```python
from build123d import *

# Parameters (mm, degrees)
F0_R     = 15
F1_DEPTH = 50
F2_R     = 25
F3_DEPTH = 5
F4_R     = 3
F5_DEPTH = 60


with BuildPart() as f1:
    # F0 (on Top) → F1 (new body)
    with BuildSketch(Plane.XY):
        Circle(F0_R)
    extrude(amount=F1_DEPTH)

    # F2 (on Top) → F3 (join)
    with BuildSketch(Plane.XY):
        Circle(F2_R)
    extrude(amount=F3_DEPTH)


with BuildPart() as f5:
    # F4 (on Top) → F5 (new body)
    with BuildSketch(Plane.XY):
        Circle(F4_R)
    extrude(amount=F5_DEPTH)


with BuildPart() as f1_1:
    add(f1.part)

    # F6: cut F5
    add(f5.part, mode=Mode.SUBTRACT)


solid = f1_1.part
```
Input: part model. Units: mm. Frame: model coordinates. Round coordinates to 2 decimals unless told otherwise and drop trailing zeros. Loops run counter-clockwise (first coordinate to the right, second up) from the corner with the lowest first, then second, coordinate; pieces in that order, holes last. Notation, with made-up numbers: (16, -5.75) -> (27, -5.75) arc R30 ccw to (27, 20.25) -> close; hole circle Ø11 at (13, 72.25). An arc over 180 degrees is marked (long way). One line per item, written item: value.
(1) Pin query (flat end, axial travel): pin 1 (6 mm diameter, centred on x = 11, z = 24.5, fed in from -Y); pin 2 (1 mm diameter, centred on x = 10.5, z = 42, fed in from +Y); pin 3 (6 mm diameter, centred on y = 1.5, z = 34.5, fed in from -X). Return the tip coordinate at first contact, or that it passes through.
Geometry check:
pin 1: y = -12.69
pin 2: y = 11.18
pin 3: x = -15
(2) Material intervals for line 1 (X direction, y = 0, z = 16.5); line 2 (X direction, y = -2, z = 17), sorted ascending. Write a range as [from, to].
Geometry check:
line 1: [-15, -3], [3, 15]
line 2: [-14.87, -2.24], [2.24, 14.87]
(3) Section A-A (x = 0). Return the cut outline in (y, z).
Geometry check:
outline: (-25, 0) -> (-3, 0) -> (-3, 50) -> (-15, 50) -> (-15, 5) -> (-25, 5) -> close; (3, 0) -> (25, 0) -> (25, 5) -> (15, 5) -> (15, 50) -> (3, 50) -> close
(4) Section C-C (z = 35). Return the cut outline in (x, y).
Geometry check:
outline: circle Ø30 at (0, 0); hole circle Ø6 at (0, 0)
(5) Section D-D (y = -13). Return the cut outline in (x, z), plus the area to 3 significant figures.
Geometry check:
outline: (-21.35, 0) -> (21.35, 0) -> (21.35, 5) -> (7.48, 5) -> (7.48, 50) -> (-7.48, 50) -> (-7.48, 5) -> (-21.35, 5) -> close
area: 887 mm2
(6) Mould query, pull axis Y, two halves, no side actions, for faces 1 (the face through (-3, 0, 25)), 2 (the face through (11, -11, 5)), 3 (the face through (-14.985, 0.66, 27.185)). Classes: pulls with the +Y half, pulls with the -Y half, needs draft (parallel to the pull), parting line crosses it, or undercut.
Geometry check:
face 1: undercut
face 2: needs draft
face 3: parting line crosses it
